from build123d import *

# Parameters (mm, degrees)
SKETCH1_W           = 127
SKETCH1_H           = 114.3
SKETCH1_R           = 2.4892
SKETCH1_R_2         = 14.2875
BOSS_EXTRUDE1_DEPTH = 1.143
FILLET1_R           = 6.35


with BuildPart() as part:
    # Sketch1 → Boss-Extrude1 (new, symmetric)
    with BuildSketch(Plane.XY):
        with Locations((63.5, 57.15)):
            Rectangle(SKETCH1_W, SKETCH1_H)
        with Locations((45.6692, 82.55)):
            Circle(SKETCH1_R, mode=Mode.SUBTRACT)
        with Locations((45.6692, 57.15)):
            Circle(SKETCH1_R_2, mode=Mode.SUBTRACT)
        with Locations((45.6692, 31.75)):
            Circle(SKETCH1_R, mode=Mode.SUBTRACT)
        with Locations((101.6, 107.95)):
            Circle(SKETCH1_R, mode=Mode.SUBTRACT)
        with Locations((101.6, 57.15)):
            Circle(SKETCH1_R_2, mode=Mode.SUBTRACT)
        with Locations((101.6, 6.35)):
            Circle(SKETCH1_R, mode=Mode.SUBTRACT)
    extrude(amount=BOSS_EXTRUDE1_DEPTH, both=True)

    # Fillet1
    fillet1_edges = [part.edges().sort_by_distance(p)[0] for p in [
        (0, 114.3, 0),
        (127, 114.3, 0),
        (127, 0, 0),
        (0, 0, 0),
    ]]
    fillet(fillet1_edges, radius=FILLET1_R)


solid = part.part
CAD build for the part. Positions are in the model's coordinates, mm. Round coordinates to 2 decimals unless told otherwise and drop trailing zeros. Loops run counter-clockwise (first coordinate to the right, second up) from the corner with the lowest first, then second, coordinate; pieces in that order, holes last. Notation, with made-up numbers: (68, 59.5) - (118, 59.5) arc R22 cw to (118, 66.5) - close; hole circle Ø9 at (-34.5, 12.5). An arc over 180 degrees is marked (long way). Put each result on its own line as item: value.
1. Slice it at B-B on x = 101.6. List the corners of the cut face in (y, z), and give its area (3 significant figures).
Geometry check:
outline: (0, -1.14) - (3.86, -1.14) - (3.86, 1.14) - (0, 1.14) - close; (8.84, -1.14) - (42.86, -1.14) - (42.86, 1.14) - (8.84, 1.14) - close; (71.44, -1.14) - (105.46, -1.14) - (105.46, 1.14) - (71.44, 1.14) - close; (110.44, -1.14) - (114.3, -1.14) - (114.3, 1.14) - (110.44, 1.14) - close
area: 173 mm²
2. Two-plate mould, pull along X, no slides. Class faces 1 (the flat face through (63, 58, 1.143)), 2 (the cylindrical face through (103.9, 5.4, 0)), 3 (the cylindrical face through (125.19, 112.39, -0.02)): released by +X, released by -X, zero draft, split by the parting line, or undercut.
Geometry check:
face 1: zero draft
face 2: undercut
face 3: released by +X
3. Slice it at A-A on y = 82.55. List the corners of the cut face in (x, z).
Geometry check:
outline: (0, -1.14) - (43.18, -1.14) - (43.18, 1.14) - (0, 1.14) - close; (48.16, -1.14) - (127, -1.14) - (127, 1.14) - (48.16, 1.14) - close
4. Slice it at C-C on y = 57.15. List the corners of the cut face in (x, z).
Geometry check:
outline: (0, -1.14) - (31.38, -1.14) - (31.38, 1.14) - (0, 1.14) - close; (59.96, -1.14) - (87.31, -1.14) - (87.31, 1.14) - (59.96, 1.14) - close; (115.89, -1.14) - (127, -1.14) - (127, 1.14) - (115.89, 1.14) - close
5. Wall check: line 1 (Y direction, x = 101.6, z = -0.5); line 2 (Y direction, x = 41.5, z = 0.45); line 3 (X direction, y = 62.5, z = 0.6). Give the ranges that are in metal, low to high.
Geometry check:
line 1: 0 to 3.86, 8.84 to 42.86, 71.44 to 105.46, 110.44 to 114.3
line 2: 0 to 43.48, 70.82 to 114.3
line 3: 0 to 32.42, 58.92 to 88.35, 114.85 to 127
6. Pin check, flat tips, straight feed: P1, Ø4, axis at x = 101.6, y = 6.35, coming from the -Z side; P2, Ø8, axis at x = 101.6, y = 107.95, coming from the -Z side. Stop position of each tip, or through.
Geometry check:
P1: through
P2: z = -1.14
7. Slice it at D-D on z = -0.7. Give the number of separate pieces and of enclosed holes in the cut face, and give its area (3 significant figures).
Geometry check:
separate pieces: 1
enclosed holes: 6
area: 13,100 mm²
